Model file for the job. Use its own axes, mm. A direction names the side the tool comes from. Round coordinates to 2 decimals unless told otherwise and drop trailing zeros. Order: outer loops, then holes, each group sorted by start corner. A loop starts at its lowest first (then second) coordinate and runs counter-clockwise, first axis right, second up. Notation, with made-up numbers: (-5.5, 42.5) - (49.5, 42.5) arc R24 cw to (49.5, 77.5) - close; hole circle Ø6 at (-19, 39). An arc over 180 degrees is marked (long way). Put each result on its own line as item: value. Start each with the question number.
Item 1: Which spindle directions (+Z, -Z, +X, -X, +Y, -Y) get a long thin tool onto all of the face, cutting with end or side? Do faces 4 (the face through (-58, 0, 27.94)), 5 (the face through (-80, -8.529, 26)). Say none if no direction does.
Item 2: Saw through at D-D on x = -77. List the corners of the cut face in (y, z).
Item 3: Saw through at B-B on z = 25.75. List the corners of the cut face in (x, y), plus the area to 3 significant figures.
Item 4: Probe probe 1 along Y at (x, z) = (-85, 24); probe 2 along Z at (x, y) = (-75, 0.5); probe 3 along Y at (x, z) = (-81, 26.25). List the from-to ranges inside material, lowest first.
Item 5: Mould opens along Y. For faces 1 (the face through (-78, 0, 23.114)), 2 (the face through (-89.452, 0.213, 13.774)), 3 (the face through (-61.95, 23.845, 13.774)) say: pulls with the +Y half, pulls with the -Y half, needs draft (parallel to the pull), parting line crosses it, or undercut.
Item 6: Saw through at C-C on y = 1.5. List the corners of the cut face in (x, z).
Item 7: Pin check, flat tips, straight feed: pin 1 Ø1.5 at (x, z) = (-57, 18) entering from +Y; pin 2 Ø8 at (y, z) = (-20, 18) entering from -X; pin 3 Ø6 at (y, z) = (26.5, 19.5) entering from +X. Stop position of each tip, or through.
Item 8: Saw through at A-A on x = -45.5. List the corners of the cut face in (y, z), plus the area to 3 significant figures.
```python
from build123d import *

# Parameters (mm, degrees)
F1_DEPTH = 27.94
F2_W     = 27.048528
F2_H     = 17.018
F3_DEPTH = 4.826
F4_R     = 2.54


with BuildPart() as f1:
    # F0 (on Top) → F1 (new body)
    with BuildSketch(Plane.XY):
        with BuildLine():
            ThreePointArc((-25.211154, -43.172467), (-49.99464, -0.013258), (-25.234047, 43.15909))
            Line((-25.234047, 43.15909), (-81.138089, 13.751116))
            ThreePointArc((-81.138089, 13.751116), (-89.453911, -0.023722), (-81.130784, -13.794148))
            Line((-81.130784, -13.794148), (-25.211154, -43.172467))
        make_face()
    extrude(amount=F1_DEPTH)

    # F2 (on face) → F3 (cut)
    with BuildSketch(Plane.XY.offset(27.94)):
        with BuildLine():
            Line((-73.894091, 8.489404), (-73.894091, -8.528596))
            ThreePointArc((-73.894091, -8.528596), (-65.385091, -0.019596), (-73.894091, 8.489404))
        make_face()
        with Locations((-87.418355, -0.019596)):
            Rectangle(F2_W, F2_H)
    extrude(amount=-F3_DEPTH, mode=Mode.SUBTRACT)

    # F4
    f4_edges = [f1.edges().sort_by_distance(p)[0] for p in [
        (-25.211154, -43.172467, 13.97),
        (-25.234047, 43.15909, 13.97),
    ]]
    fillet(f4_edges, radius=F4_R)


solid = f1.part
```
Results found:
1. face 4: +Z, +X, -X, +Y, -Y
1. face 5: +Z, -X
2. outline: (-15.96, 0) - (15.93, 0) - (15.93, 27.94) - (8.49, 27.94) - (8.49, 23.11) - (-8.53, 23.11) - (-8.53, 27.94) - (-15.96, 27.94) - close
3. outline: (-86.92, -8.53) arc R15.56 ccw to (-81.13, -13.79) - (-43.27, -33.68) arc R2.54 ccw to (-40.06, -29.91) arc R49.99 cw to (-40.07, 29.89) arc R2.54 ccw to (-43.29, 33.66) - (-81.14, 13.75) arc R15.56 ccw to (-86.92, 8.49) - (-73.89, 8.49) arc R8.51 cw to (-73.89, -8.53) - close
3. area: 1,410 mm²
4. probe 1: y = -10.92 to -8.53, 8.49 to 10.88
4. probe 2: z = 0 to 23.11
4. probe 3: y = -13.86 to -8.53, 8.49 to 13.82
5. face 1: undercut
5. face 2: parting line crosses it
5. face 3: pulls with the +Y half
6. outline: (-89.38, 0) - (-49.97, 0) - (-49.97, 27.94) - (-65.52, 27.94) - (-65.52, 23.11) - (-89.38, 23.11) - close
7. pin 1: stops at y = 26.84
7. pin 2: stops at x = -76.93
7. pin 3: stops at x = -40.36
8. outline: (-32.51, 0) - (-20.72, 0) - (-20.72, 27.94) - (-32.51, 27.94) - close; (20.72, 0) - (32.5, 0) - (32.5, 27.94) - (20.72, 27.94) - close
8. area: 659 mm²
